Part model, mm, in its own coordinate system. A direction names the side the tool comes from. Give positions to 0.01 mm unless a question says otherwise; leave off trailing zeros. Order: outer loops, then holes, each group sorted by start corner. A loop starts at its lowest first (then second) coordinate and runs counter-clockwise, first axis right, second up. Notation, with made-up numbers: (-37.75, 31.25) - (5.25, 31.25) arc R34 ccw to (5.25, 69.25) - close; hole circle Ø5 at (-31.5, 29). An arc over 180 degrees is marked (long way). Use one line per item in the form item = value. Start each with the question number.
1. Pull direction X, two halves, no side cores. Call faces 5 (the face through (-0.14, -1.565, -29.462)), 6 (the face through (-2, 3.175, 1)), 7 (the face through (-18.335, -1.61, 9.722)): +X half, -X half, draft (parallel to the pull), parting line (faces both ways), or undercut.
2. Band-saw the part on B-B, the plane z = 0. List the corners of the cut face in (x, y) (3 decimals).
3. Drill centre lines: line 1 (Z direction, x = 0, y = 1.5); line 2 (Y direction, x = 23, z = 10.5) (3 decimals); line 3 (X direction, y = -0.5, z = -0.5). Where is each one in solid material? Low to high.
4. Pin check, flat tips, straight feed: P1, Ø3, axis at y = -0.5, z = -18, coming from the +X side; P2, Ø2, axis at x = -10.5, y = 1.5, coming from the +Z side; P3, Ø1.5, axis at y = -0.5, z = 9, coming from the +X side; P4, Ø3, axis at x = -20.02, z = 11.56, coming from the +Y side. Stop position of each tip, or through.
5. Band-saw the part on A-A, the plane x = 0. List the corners of the cut face in (y, z) (3 decimals).
6. Band-saw the part on C-C, the plane y = -2. List the corners of the cut face in (x, z) (3 decimals), plus the area to 3 significant figures.
7. Tool access for faces 1 (the face through (-0.03, 1.61, -16.764)), 2 (the face through (-16.993, 1.565, 4.068)), 3 (the face through (16.985, 1.565, 3.984)), 4 (the face through (-12.17, -1.37, 14.36)): list every direction of +Z, -Z, +X, -X, +Y, -Y with a clear straight run to the whole face (end or side of a thin tool).
from build123d import *

# Parameters (mm, degrees)
SKETCH1_R           = 2.0193
SKETCH1_R_2         = 2.4892
BOSS_EXTRUDE1_DEPTH = 3.175
SKETCH3_R           = 6.35
SKETCH3_R_2         = 2.4892
CUT_EXTRUDE1_DEPTH  = 3.175
CIRPATTERN1_COUNT   = 3
FILLET3_R           = 15.24
FILLET2_DEPTH       = 3.175


with BuildPart() as part:
    # Sketch1 → Boss-Extrude1 (new, symmetric)
    with BuildSketch(Plane(origin=(0, 0, 0), x_dir=(1, 0, 0), z_dir=(0, 1, 0))):
        with BuildLine():
            Line((-6.35, 0), (-6.35, 23.114))
            ThreePointArc((-6.35, 23.114), (0, 29.464), (6.35, 23.114))
            Line((6.35, 23.114), (6.35, 0))
            ThreePointArc((6.35, 0), (0, -6.35), (-6.35, 0))
        make_face()
        with Locations(Location((0, 0, 0), (0, 0, 270))):
            Circle(SKETCH1_R, mode=Mode.SUBTRACT)
        with Locations(Location((0, 23.114, 0), (0, 0, 270))):
            Circle(SKETCH1_R_2, mode=Mode.SUBTRACT)
    boss_extrude1 = extrude(amount=BOSS_EXTRUDE1_DEPTH, both=True)

    # Sketch3 → Cut-Extrude1 (cut)
    with BuildSketch(Plane(origin=(0, 3.175, 0), x_dir=(1, 0, 0), z_dir=(0, 1, 0))):
        with Locations((0, 23.114)):
            Circle(SKETCH3_R)
        with Locations(Location((0, 23.114, 0), (0, 0, 270))):
            Circle(SKETCH3_R_2, mode=Mode.SUBTRACT)
    cut_extrude1 = extrude(amount=-CUT_EXTRUDE1_DEPTH, mode=Mode.SUBTRACT)

    # CirPattern1: Boss-Extrude1, Cut-Extrude1 ×3 about axis
    cirpattern1_axis = Axis((0, 0, 0), (0, 1, 0))
    add([boss_extrude1.rotate(cirpattern1_axis, i * 360 / CIRPATTERN1_COUNT) for i in range(1, CIRPATTERN1_COUNT)])
    add([cut_extrude1.rotate(cirpattern1_axis, i * 360 / CIRPATTERN1_COUNT) for i in range(1, CIRPATTERN1_COUNT)], mode=Mode.SUBTRACT)

    # Fillet3
    fillet3_edges = [part.edges().sort_by_distance(p)[0] for p in [
        (-6.35, 0, -3.666174209),
        (6.35, 0, -3.666174209),
        (0, 0, 7.332348419),
    ]]
    fillet(fillet3_edges, radius=FILLET3_R)

    # Fillet2: read off the stored shape, not the designer's step
    # Fillet2 outline → Fillet2 (cut)
    with BuildSketch(Plane(origin=(0, 0, 0), x_dir=(1, 0, 0), z_dir=(0, 1, 0))):
        with BuildLine():
            ThreePointArc((15.41518125, -1.567610625), (16.989288832, -4.025929604), (15.890891228, -6.730494188))
            ThreePointArc((15.890891228, -6.730494188), (19.434687828, -5.233784835), (23.192311183, -6.057738686))
            Line((23.192311183, -6.057738686), (15.41518125, -1.567610625))
        make_face()
        with BuildLine():
            ThreePointArc((16.842311183, -17.056261314), (14.249934539, -14.214040956), (13.774224561, -10.396668398))
            ThreePointArc((13.774224561, -10.396668398), (11.981201728, -12.700190919), (9.06518125, -12.566133253))
            Line((9.06518125, -12.566133253), (16.842311183, -17.056261314))
        make_face()
        with BuildLine():
            ThreePointArc((-9.06518125, -12.566133253), (-11.981201728, -12.700190919), (-13.774224561, -10.396668398))
            ThreePointArc((-13.774224561, -10.396668398), (-14.249934539, -14.214040956), (-16.842311183, -17.056261314))
            Line((-16.842311183, -17.056261314), (-9.06518125, -12.566133253))
        make_face()
        with BuildLine():
            ThreePointArc((-23.192311183, -6.057738686), (-19.434687828, -5.233784835), (-15.890891228, -6.730494188))
            ThreePointArc((-15.890891228, -6.730494188), (-16.989288832, -4.025929604), (-15.41518125, -1.567610625))
            Line((-15.41518125, -1.567610625), (-23.192311183, -6.057738686))
        make_face()
        with BuildLine():
            ThreePointArc((-6.35, 14.133743879), (-5.008087105, 16.726120523), (-2.116666667, 17.127162586))
            ThreePointArc((-2.116666667, 17.127162586), (-5.184753289, 19.447825791), (-6.35, 23.114))
            Line((-6.35, 23.114), (-6.35, 14.133743879))
        make_face()
        with BuildLine():
            ThreePointArc((2.116666667, 17.127162586), (5.008087105, 16.726120523), (6.35, 14.133743879))
            Line((6.35, 14.133743879), (6.35, 23.114))
            ThreePointArc((6.35, 23.114), (5.184753289, 19.447825791), (2.116666667, 17.127162586))
        make_face()
    extrude(amount=FILLET2_DEPTH, mode=Mode.SUBTRACT)


solid = part.part
From the geometry:
q1.face_5 = parting line
q1.face_6 = draft
q1.face_7 = undercut
q2.outline = (-12.822, -3.175) - (-2.019, -3.175) - (-2.019, 3.175) - (-12.822, 3.175) - close; (2.019, -3.175) - (12.822, -3.175) - (12.822, 3.175) - (2.019, 3.175) - close
q3.line_1 = -16.76 to -2.02, 2.02 to 9.69
q3.line_2 = -3.175 to 0
q3.line_3 = -12.15 to -1.96, 1.96 to 12.15
q4.P1 = 6.35
q4.P2 = 12.99
q4.P3 = 26.1
q4.P4 = through
q5.outline = (-3.175, -29.464) - (0, -29.464) - (0, -25.603) - (-3.175, -25.603) - close; (-3.175, -20.625) - (0, -20.625) - (0, -16.764) - (3.175, -16.764) - (3.175, -2.019) - (-3.175, -2.019) - close; (-3.175, 2.019) - (3.175, 2.019) - (3.175, 9.69) - (-3.175, 9.69) - close
q6.outline = (-23.192, 6.058) - (-13.97, 0.733) arc R15.24 cw to (-6.35, -12.465) - (-6.35, -23.114) arc R6.35 ccw to (6.35, -23.114) - (6.35, -12.465) arc R15.24 cw to (13.97, 0.733) - (23.192, 6.058) arc R6.35 ccw to (16.842, 17.056) - (7.62, 11.732) arc R15.24 cw to (-7.62, 11.732) - (-16.842, 17.056) arc R6.35 ccw to start; hole circle Ø4.978 at (-20.017, 11.557); hole circle Ø4.978 at (0, -23.114); hole circle Ø4.039 at (0, 0); hole circle Ø4.978 at (20.017, 11.557)
q6.area = 967 mm²
q7.face_1 = -Z, +Y
q7.face_2 = -X, +Y
q7.face_3 = +X, +Y
q7.face_4 = +Z, +Y, -Y
